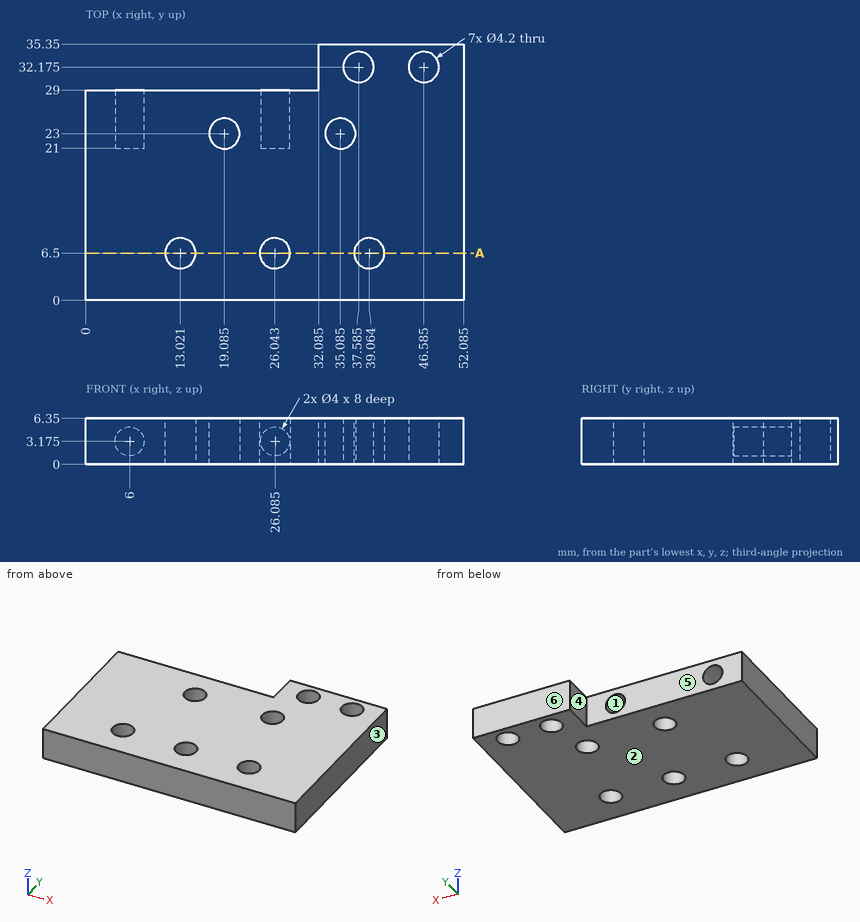
Input: dimensioned drawing with shaded views. Units: mm. Origin: part minimum x, y, z. A direction names the side the tool comes from. Round coordinates to 2 decimals unless told otherwise and drop trailing zeros. Answer as a JSON object with one key per item and string values. Group by question number.
(1) Material intervals for probe 1 along X at (y, z) = (27, 3.25) (1 decimal); probe 2 along X at (y, z) = (24, 5.75) (1 decimal); probe 3 along Y at (x, z) = (26, 3.75), sorted ascending. Write a range as from..to.
(2) Draft query along X for the marked faces 1, 2, 3 and 4. Return one class per face: released by +X, released by -X, zero draft, split by the parting line, or undercut.
(3) Reachability of the marked faces 5 and 6 from +Z, -Z, +X, -X, +Y, -Y: full face, straight path, thin tool, end or side. Return the list, or none.
(4) Cut plane A-A (y = 6.5). Count the separate pieces of the cut face and the enclosed holes in it, then the cut area to 3 significant figures.
(5) Pin query (flat end, axial travel): P1, Ø2.5, axis at x = 6, z = 3.175, coming from the +Y side; P2, Ø1.9, axis at x = 18.5, z = 4, coming from the +Y side; P3, Ø2.5, axis at x = 37.59, y = 32.17, coming from the -Z side. Return the tip coordinate at first contact, or that it passes through.
Here are the results:
{
 "1": {"probe 1": "x = 0..4, 8..24.1, 28.1..52.1", "probe 2": "x = 0..17.2, 20.9..33.2, 36.9..52.1", "probe 3": "y = 0..4.4, 8.6..21"},
 "2": {"face 1": "undercut", "face 2": "zero draft", "face 3": "released by +X", "face 4": "released by -X"},
 "3": {"face 5": "+Z, -Z, -X, +Y", "face 6": "+Z, -Z, +X, -X, +Y"},
 "4": {"separate pieces": "4", "enclosed holes": "0", "area": "251 mm^2"},
 "5": {"P1": "stops at y = 21", "P2": "stops at y = 29", "P3": "passes through"}
}
